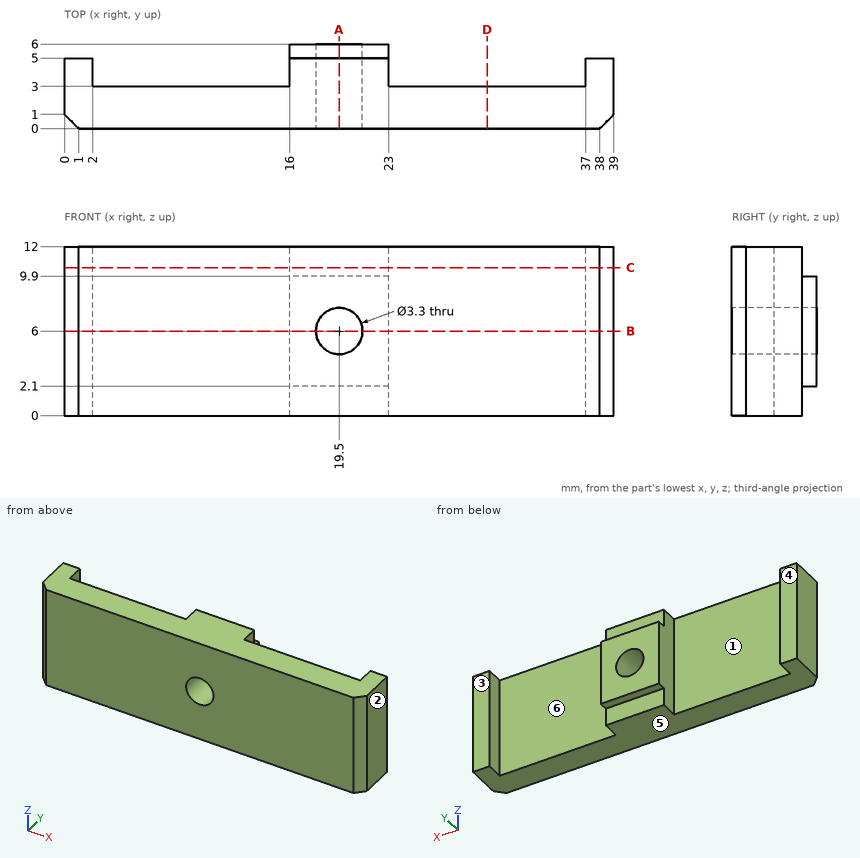
Can you work these out from the drawing? Everything is in mm from the part's minimum corner. A direction names the side the tool comes from. Coordinates: 2 decimals unless noted, no trailing zeros. Loops run counter-clockwise (first coordinate to the right, second up) from the corner with the lowest first, then second, coordinate; pieces in that order, holes last. Notation, with made-up numbers: M 30.5,26.25 L 36.5,26.25 A28 ccw 36.5,44.25 Z; hole C 34.25,32.5 d3. An arc over 180 degrees is marked long. Put each result on its own line as item: value. Start each with the question number.
(1) Thinking about a two-plate mould opening in X: for the marked faces 1, 2 and 3, which applies, pulls with the +X half, pulls with the -X half, needs draft (parallel to the pull), parting line crosses it, or undercut?
(2) For the marked faces 4, 5 and 6, which set-ups out of +Z, -Z, +X, -X, +Y, -Y let a thin tool reach every point of the face, with its end or its side?
(3) Suppose I cut it at A-A on x = 19.5. Please give me the cut outline in (y, z), then the cut area to 3 significant figures.
(4) Suppose I cut it at C-C on z = 10.5. Please give me the cut outline in (x, y), then the cut area to 3 significant figures.
(5) Suppose I cut it at D-D on x = 30. Please give me the cut outline in (y, z), then the cut area to 3 significant figures.
(6) I need wall thicknesses on line 1 (X direction, y = 4, z = 6); line 2 (X direction, y = 3.5, z = 1.75); line 3 (Z direction, x = 19.5, y = 1.35). Which ranges of each line are inside material? Lowest first, please. Write a range as from..to.
(7) Will these pins go through, and if not, where does the flat tip stop? P1, Ø1, axis at y = 3.5, z = 4.5, coming from the -X side; P2, Ø0.6, axis at x = 21, z = 10.5, coming from the +Y side; P3, Ø0.8, axis at x = 18.5, y = 5.5, coming from the +Z side.
(8) Suppose I cut it at B-B on z = 6. Please give me the cut outline in (x, y), then the cut area to 3 significant figures.
Solutions:
1. face 1: undercut
1. face 2: pulls with the +X half
1. face 3: needs draft
2. face 4: +Z, -Z, -X, +Y
2. face 5: -Z, +X, -X, +Y, -Y
2. face 6: +Z, -Z, +Y
3. outline: M 0,0 L 5,0 L 5,2.1 L 6,2.1 L 6,4.35 L 0,4.35 Z; M 0,7.65 L 6,7.65 L 6,9.9 L 5,9.9 L 5,12 L 0,12 Z
3. area: 48.0 mm2
4. outline: M 0,1 L 1,0 L 38,0 L 39,1 L 39,5 L 37,5 L 37,3 L 23,3 L 23,5 L 16,5 L 16,3 L 2,3 L 2,5 L 0,5 Z
4. area: 138 mm2
5. outline: M 0,0 L 3,0 L 3,12 L 0,12 Z
5. area: 36.0 mm2
6. line 1: x = 0..2, 16..17.85, 21.15..23, 37..39
6. line 2: x = 0..2, 16..23, 37..39
6. line 3: z = 0..4.35, 7.65..12
7. P1: stops at x = 0
7. P2: stops at y = 5
7. P3: stops at z = 9.9
8. outline: M 0,1 L 1,0 L 17.85,0 L 17.85,6 L 16,6 L 16,3 L 2,3 L 2,5 L 0,5 Z; M 21.15,0 L 38,0 L 39,1 L 39,5 L 37,5 L 37,3 L 23,3 L 23,6 L 21.15,6 Z
8. area: 125 mm2
